Design review of the part built by this model. Coordinates are the model's own, in mm. Face numbers are marked on the shaded views. Coordinates: 2 decimals unless noted, no trailing zeros. Loops run counter-clockwise (first coordinate to the right, second up) from the corner with the lowest first, then second, coordinate; pieces in that order, holes last.
Q1. Draft analysis for pull direction Z (two halves, no side actions). For the marked faces 1 and 2, state which applies: released by +Z, released by -Z, zero draft, split by the parting line, or undercut.
Q2. Add section A-A on y = -102535.5. Give the boundary of the cut face in (x, z), and give its area (3 significant figures).
Q3. Wall thickness on probe 1 along Z at (x, y) = (1581, -102535.25); probe 2 along Y at (x, z) = (1453.5, -28917); probe 3 along Z at (x, y) = (1364.5, -102526.5): over which ranges is each line inside the solid? List them lowest first.
Q4. For P1, Ø6, axis at x = 1214.5, z = -28906.5, coming from the -Y side; P2, Ø2, axis at x = 1414.5, z = -28921, coming from the -Y side, all flat-tipped, find the tip position at first contact; note any pin that passes through.
Q5. Add section B-B on x = 1413. Give the boundary of the cut face in (y, z), and give its area (3 significant figures).
Q6. Add section C-C on z = -28910. Give the boundary of the cut face in (x, y).
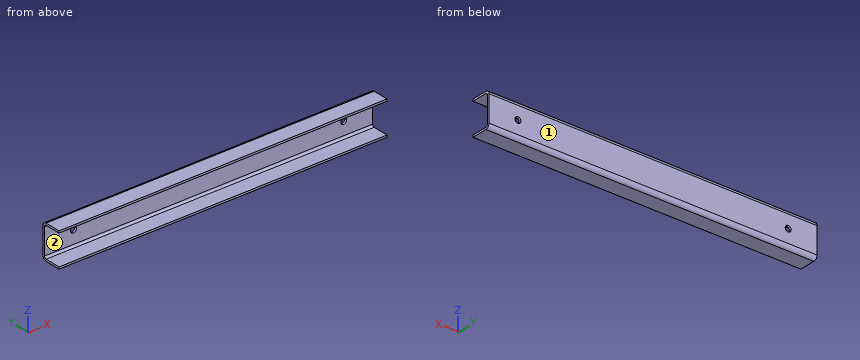
```python
from build123d import *

# Parameters (mm, degrees)
SKETCH1_W               = 500
SKETCH1_H               = 40
SKETCH1_R               = 4.5
BASE_FLANGE1_DEPTH      = 3
EDGE_FLANGE1_DEPTH      = 500
EDGE_FLANGE1_BEND_DEPTH = 500


# Sheet-metal steps are written as plain solids
with BuildPart() as part:
    # Sketch1 → Base-Flange1 (new body)
    with BuildSketch(Plane(origin=(1355.32335997, -102522.563627841, -30605.108385113), x_dir=(1, 0, 0), z_dir=(0, 1, 0))):
        with Locations((0.368301387, -1705.033559341)):
            Rectangle(SKETCH1_W, SKETCH1_H)
        with Locations(Location((-205.631698613, -1705.033559341, 0), (0, 0, 270))):
            Circle(SKETCH1_R, mode=Mode.SUBTRACT)
        with Locations(Location((206.368301387, -1705.033559341, 0), (0, 0, 270))):
            Circle(SKETCH1_R, mode=Mode.SUBTRACT)
    extrude(amount=-BASE_FLANGE1_DEPTH)

    # Edge-Flange1 section (across the edge) → Edge-Flange1 (add)
    with BuildSketch(Plane(origin=(1605.691661356, -102525.563627841, -28877.074825771), x_dir=(0, 0, -1), z_dir=(-1, 0, 0))):
        with BuildLine():
            Line((-3, 3), (-3, 27))
            Line((-3, 27), (0, 27))
            Line((0, 27), (0, 3))
            ThreePointArc((0, 3), (0.878679656, 0.878679656), (3, 0))
            Line((3, 0), (3, -3))
            ThreePointArc((3, -3), (-1.242640687, -1.242640687), (-3, 3))
        make_face()
    extrude(amount=EDGE_FLANGE1_DEPTH)

    # Edge-Flange1 section 2 (across the edge) → Edge-Flange1 bend (add)
    with BuildSketch(Plane(origin=(1105.691661356, -102525.563627841, -28923.074825771), x_dir=(0, 0, 1), z_dir=(1, 0, 0))):
        with BuildLine():
            Line((-3, 3), (-3, 27))
            Line((-3, 27), (0, 27))
            Line((0, 27), (0, 3))
            ThreePointArc((0, 3), (0.878679656, 0.878679656), (3, 0))
            Line((3, 0), (3, -3))
            ThreePointArc((3, -3), (-1.242640687, -1.242640687), (-3, 3))
        make_face()
    extrude(amount=EDGE_FLANGE1_BEND_DEPTH)


solid = part.part
```
Entries:
1. face 1: zero draft
1. face 2: undercut
2. outline: (1105.69, -28926.07) - (1605.69, -28926.07) - (1605.69, -28923.07) - (1105.69, -28923.07) - close; (1105.69, -28877.07) - (1605.69, -28877.07) - (1605.69, -28874.07) - (1105.69, -28874.07) - close
2. area: 3,000 mm2
3. probe 1: z = -28926.07 to -28923.07, -28877.07 to -28874.07
3. probe 2: y = -102525.56 to -102522.56
3. probe 3: z = -28925.71 to -28922.25, -28877.9 to -28874.44
4. P1: stops at y = -102525.56
4. P2: stops at y = -102526.26
5. outline: (-102552.56, -28926.07) - (-102528.56, -28926.07) arc R6 ccw to (-102522.56, -28920.07) - (-102522.56, -28880.07) arc R6 ccw to (-102528.56, -28874.07) - (-102552.56, -28874.07) - (-102552.56, -28877.07) - (-102528.56, -28877.07) arc R3 cw to (-102525.56, -28880.07) - (-102525.56, -28920.07) arc R3 cw to (-102528.56, -28923.07) - (-102552.56, -28923.07) - close
5. area: 306 mm2
6. outline: (1105.69, -102525.56) - (1605.69, -102525.56) - (1605.69, -102522.56) - (1105.69, -102522.56) - close
